Work out the finished part from the listing and answer in its coordinate system (mm). A direction names the side the tool comes from. Round coordinates to 2 decimals unless told otherwise and drop trailing zeros. Order: outer loops, then holes, each group sorted by start corner. A loop starts at its lowest first (then second) coordinate and runs counter-clockwise, first axis right, second up. Notation, with made-up numbers: (62.25, 2) -> (79.25, 2) arc R30 cw to (79.25, 38) -> close; hole circle Ø8 at (-30.5, -17.5). An arc over 180 degrees is marked (long way). Use a Markdown table: item, result. Add a question column.
Item 1: A tool of negligible diameter and unlimited length cuts with its end or side. For faces 4 (the flat face through (-11, -0.635, 2)), 5 (the flat face through (-11, -8.255, 2)), 6 (the flat face through (-17.78, -4, 0)), from which of +Z, -Z, +X, -X, +Y, -Y can it reach the whole face along a straight path? Write none if from no direction.
Item 2: Find the intervals of material crossed by L1, parallel to X at y = 5.5, z = 2; L2, parallel to X at y = -3, z = 2.75; L3, parallel to Y at x = 169.5, z = -4.75, in increasing order. Write a range as [from, to].
Item 3: A cutting plane is placed at D-D, the plane x = 61. Determine the outline of the cut face in (y, z) (3 decimals).
Item 4: A cutting plane is placed at B-B, the plane z = 0. Give the number of separate pieces and of enclosed holes in the cut face, plus the area to 3 significant figures.
Item 5: A cutting plane is placed at A-A, the plane y = -3. Determine the outline of the cut face in (x, z) (3 decimals), plus the area to 3 significant figures.
Item 6: Flat-ended cylindrical pins translate along their axes: P1, Ø8, axis at x = 7, z = -3.5, coming from the -Y side; P2, Ø9, axis at x = -12, z = -1.5, coming from the -Y side; P3, Ø1.5, axis at x = 145, z = 3, coming from the +Y side. Find the tip coordinate at first contact, or state that the pin passes through.
Item 7: For a pull along Z with two mould halves and no side action, classify faces 1 (the flat face through (-16.4, 8.255, 2.3)), 2 (the flat face through (79, 0, -9.525)), 3 (the cylindrical face through (-10.72, 4.39, 0.95)) as +Z half, -Z half, draft (parallel to the pull), parting line (faces both ways), or undercut.
from build123d import *

# Parameters (mm, degrees)
F0_R     = 7.9375
F1_DEPTH = 9.525
F3_D     = 6.35


with BuildPart() as f1:
    # F0 (on Top) → F1 (new body, symmetric)
    with BuildSketch(Plane.XY):
        with BuildLine():
            ThreePointArc((-9.50381, 0.635), (0.317677, 9.519701), (9.525, 0))
            ThreePointArc((9.525, 0), (0.317677, -9.519701), (-9.50381, -0.635))
            Line((-9.50381, -0.635), (-12.7, -0.635))
            Line((-12.7, -0.635), (-17.78, -0.635))
            Line((-17.78, -0.635), (-17.78, -8.255))
            Line((-17.78, -8.255), (-9.720665, -8.255))
            ThreePointArc((-9.720665, -8.255), (-5.355366, -11.560078), (0, -12.7))
            Line((0, -12.7), (168.275, -11.1125))
            ThreePointArc((168.275, -11.1125), (179.28316, 0), (168.275, 11.1125))
            Line((168.275, 11.1125), (0, 12.7))
            ThreePointArc((0, 12.7), (-5.355366, 11.560078), (-9.720665, 8.255))
            Line((-9.720665, 8.255), (-17.78, 8.255))
            Line((-17.78, 8.255), (-17.78, 0.635))
            Line((-17.78, 0.635), (-12.7, 0.635))
            Line((-12.7, 0.635), (-9.50381, 0.635))
        make_face()
        with Locations((168.275, 0)):
            Circle(F0_R, mode=Mode.SUBTRACT)
    extrude(amount=F1_DEPTH, both=True)

    # F3 (through all)
    with Locations(Plane(origin=(0, 8.255, 0), x_dir=(-1, 0, 0), z_dir=(0, 1, 0))):
        with Locations((13.750333, 0)):
            Hole(F3_D / 2)


solid = f1.part
Reported:
| question | item | result |
|---|---|---|
| 1 | face 4 | +Z, -Z, -X |
| 1 | face 5 | +Z, -Z, -X, -Y |
| 1 | face 6 | +Z, -Z, -X, +Y, -Y |
| 2 | L1 | [-17.78, -16.22], [-11.28, -7.78], [7.78, 162.55], [174, 177.83] |
| 2 | L2 | [-17.78, -15.34], [-12.16, -9.04], [9.04, 160.93], [175.62, 178.87] |
| 2 | L3 | [-11.03, -7.84], [7.84, 11.03] |
| 3 | outline | (-12.125, -9.525) -> (12.125, -9.525) -> (12.125, 9.525) -> (-12.125, 9.525) -> close |
| 4 | separate pieces | 3 |
| 4 | enclosed holes | 1 |
| 4 | area | 3,960 mm² |
| 5 | outline | (-17.78, -9.525) -> (-9.04, -9.525) -> (-9.04, 9.525) -> (-17.78, 9.525) -> close; (9.04, -9.525) -> (160.926, -9.525) -> (160.926, 9.525) -> (9.04, 9.525) -> close; (175.624, -9.525) -> (178.871, -9.525) -> (178.871, 9.525) -> (175.624, 9.525) -> close; hole circle Ø6.35 at (-13.75, 0) |
| 5 | area | 3,090 mm² |
| 6 | P1 | y = -12.67 |
| 6 | P2 | y = -10.31 |
| 6 | P3 | y = 11.34 |
| 7 | face 1 | draft |
| 7 | face 2 | -Z half |
| 7 | face 3 | undercut |
